Design review of the part built by this model. Coordinates are the model's own, in mm. A direction names the side the tool comes from. Coordinates: 2 decimals unless noted, no trailing zeros. Loops run counter-clockwise (first coordinate to the right, second up) from the corner with the lowest first, then second, coordinate; pieces in that order, holes last. Notation, with made-up numbers: (-6.5, -6.5) -> (37.5, -6.5) arc R36 cw to (37.5, 32.5) -> close; hole circle Ø4 at (1.5, -15.5). An arc over 180 degrees is marked (long way). Answer as a JSON object with one key per item and string values.
```python
from build123d import *

# Parameters (mm, degrees)
SKETCH1_W           = 81.6864
SKETCH1_H           = 72.4154
BOSS_EXTRUDE1_DEPTH = 1.5748
SKETCH2_W           = 77.7
SKETCH2_H           = 56.5
BOSS_EXTRUDE2_DEPTH = 4.27
SKETCH4_R           = 1.55
CUT_EXTRUDE1_DEPTH  = 58.189442313
SKETCH3_W           = 12.7
SKETCH3_H           = 5.08
SKETCH3_W_2         = 34.071115987
BOSS_EXTRUDE3_DEPTH = 5.08
SKETCH5_W           = 11.143297124
SKETCH5_H           = 14.820585176
SKETCH5_W_2         = 5.702652661
SKETCH5_H_2         = 0.935331402
BOSS_EXTRUDE4_DEPTH = 1


with BuildPart() as part:
    # Sketch1 → Boss-Extrude1 (new body)
    with BuildSketch(Plane(origin=(0, 0, 0), x_dir=(-1, 0, 0), z_dir=(0, 0, -1))):
        with Locations((2.8568, -0.2173)):
            Rectangle(SKETCH1_W, SKETCH1_H)
    extrude(amount=BOSS_EXTRUDE1_DEPTH)

    # Sketch2 → Boss-Extrude2 (add)
    with BuildSketch(Plane(origin=(0, 0, 0), x_dir=(-1, 0, 0), z_dir=(0, 0, -1))):
        with Locations((2.85, -0.25)):
            Rectangle(SKETCH2_W, SKETCH2_H)
    extrude(amount=-BOSS_EXTRUDE2_DEPTH)

    # Sketch4 → Cut-Extrude1 (cut, through all)
    with BuildSketch(Plane(origin=(0, 0, -1.5748), x_dir=(-1, 0, 0), z_dir=(0, 0, -1))):
        with Locations((39.525, 31.8154)):
            Circle(SKETCH4_R)
        with Locations((39.525, -32.625)):
            Circle(SKETCH4_R)
        with Locations((-12.735, -32.625)):
            Circle(SKETCH4_R)
        with Locations((-33.8114, 31.8154)):
            Circle(SKETCH4_R)
    extrude(amount=-CUT_EXTRUDE1_DEPTH, mode=Mode.SUBTRACT)

    # Sketch3 → Boss-Extrude3 (add)
    with BuildSketch(Plane.XY.offset(-1.5748)):
        with Locations((19.31004682, 31.274104804)):
            Rectangle(SKETCH3_W, SKETCH3_H)
        with Locations((-17.035557993, 31.274104804)):
            Rectangle(SKETCH3_W_2, SKETCH3_H)
        with Locations((-17.035557993, -31.699250815)):
            Rectangle(SKETCH3_W_2, SKETCH3_H)
    extrude(amount=-BOSS_EXTRUDE3_DEPTH)

    # Sketch5 → Boss-Extrude4 (add)
    with BuildSketch(Plane(origin=(0, 0, -1.5748), x_dir=(-1, 0, 0), z_dir=(0, 0, -1))):
        Polygon((19.476551601, 13.535617464), (30.731281697, 2.280887368), (19.476551601, -8.973842728), (8.221821505, 2.280887368), align=None)
        with Locations((-21.419348846, -17.387032057)):
            Rectangle(SKETCH5_W, SKETCH5_H)
        with Locations((-34.20974354, -34.592993391)):
            Rectangle(SKETCH5_W_2, SKETCH5_H_2)
    extrude(amount=BOSS_EXTRUDE4_DEPTH)


solid = part.part
```
1) For faces 1 (the flat face through (-17, -29.159, -4)), 2 (the flat face through (25.66, 31, -4)), 3 (the flat face through (-25.025, 7.987, -2.068)), 4 (the flat face through (-34.071, 31, -4)), list the 3-axis set-ups (+Z, -Z, +X, -X, +Y, -Y) from which the entire face can be reached by the end or side of a thin tool; tool diameter is ignored.
Completed:
{"face 1": "-Z, +X, -X", "face 2": "-Z, +X, +Y", "face 3": "-Z, -X", "face 4": "-Z, -X, +Y, -Y"}
2) Clearance check with flat-ended pins moving along their axes: pin 1 Ø11.5 at (x, y) = (-24.5, 1.5) entering from -Z; pin 2 Ø3 at (x, z) = (-27, -4.5) entering from +Y; pin 3 Ø1 at (x, y) = (6, -16.5) entering from -Z. State where each tip first meets the part, or that it passes through.
Completed:
{"pin 1": "z = -2.57", "pin 2": "y = 33.81", "pin 3": "z = -1.57"}
3) Add section A-A, the plane x = 22.5. Give the boundary of the cut face in (y, z) (3 decimals), and give its area (3 significant figures).
Completed:
{"outline": "(-36.425, -1.575) -> (-24.797, -1.575) -> (-24.797, -2.575) -> (-9.977, -2.575) -> (-9.977, -1.575) -> (28.734, -1.575) -> (28.734, -6.655) -> (33.814, -6.655) -> (33.814, -1.575) -> (35.99, -1.575) -> (35.99, 0) -> (28, 0) -> (28, 4.27) -> (-28.5, 4.27) -> (-28.5, 0) -> (-36.425, 0) -> close", "area": "396 mm²"}
4) Add section C-C, the plane z = 1.75. Give the boundary of the cut face in (x, y), and give its area (3 significant figures).
Completed:
{"outline": "(-41.7, -28.5) -> (36, -28.5) -> (36, 28) -> (-41.7, 28) -> close", "area": "4,390 mm²"}
5) Add section B-B, the plane y = -15. Give the boundary of the cut face in (x, z), and give its area (3 significant figures).
Completed:
{"outline": "(-43.7, -1.57) -> (15.85, -1.57) -> (15.85, -2.57) -> (26.99, -2.57) -> (26.99, -1.57) -> (37.99, -1.57) -> (37.99, 0) -> (36, 0) -> (36, 4.27) -> (-41.7, 4.27) -> (-41.7, 0) -> (-43.7, 0) -> close", "area": "472 mm²"}
6) Add section D-D, the plane y = 16.5. Give the boundary of the cut face in (x, z).
Completed:
{"outline": "(-43.7, -1.57) -> (37.99, -1.57) -> (37.99, 0) -> (36, 0) -> (36, 4.27) -> (-41.7, 4.27) -> (-41.7, 0) -> (-43.7, 0) -> close"}
7) The part is to be moulded in two halves that separate along Y. For faces 5 (the flat face through (-17, -32, -6.655)), 6 (the flat face through (-2, -28.5, 2)), 7 (the flat face through (-13.9, -3.4, -2.1)), 8 (the flat face through (-2, 28, 2)), say which applies: pulls with the +Y half, pulls with the -Y half, needs draft (parallel to the pull), parting line crosses it, or undercut.
Completed:
{"face 5": "needs draft", "face 6": "pulls with the -Y half", "face 7": "undercut", "face 8": "pulls with the +Y half"}
8) Wall thickness on probe 1 along Z at (x, y) = (-37.5, 15); probe 2 along Y at (x, z) = (17, -4.25); probe 3 along Z at (x, y) = (15, -29.5): over which ranges is each line inside the solid? List them lowest first.
Completed:
{"probe 1": "-1.57 to 4.27", "probe 2": "28.73 to 33.81", "probe 3": "-1.57 to 0"}
